```python
from build123d import *

# Parameters (mm, degrees)
SKETCH1_R           = 15
BOSS_EXTRUDE1_DEPTH = 850
SKETCH3_W           = 20
SKETCH3_H           = 50
BOSS_EXTRUDE2_DEPTH = 50


with BuildPart() as part:
    # Sketch1 → Boss-Extrude1 (new body)
    with BuildSketch(Plane.XY):
        Circle(SKETCH1_R)
    extrude(amount=BOSS_EXTRUDE1_DEPTH)

    # Sketch3 → Boss-Extrude2 (add)
    with BuildSketch(Plane.XY.offset(850)):
        Rectangle(SKETCH3_W, SKETCH3_H)
    boss_extrude2 = extrude(amount=BOSS_EXTRUDE2_DEPTH)

    # Mirror1: Boss-Extrude2 across plane
    add(boss_extrude2.mirror(Plane(origin=(0, 0, 425), x_dir=(1, 0, 0), z_dir=(0, 0, -1))))


solid = part.part
```
Input: part model. Units: mm. Frame: model coordinates. A direction names the side the tool comes from. Round coordinates to 2 decimals unless told otherwise and drop trailing zeros. Loops run counter-clockwise (first coordinate to the right, second up) from the corner with the lowest first, then second, coordinate; pieces in that order, holes last.
1) Pin query (flat end, axial travel): pin 1 (3 mm diameter, centred on x = 1, z = 82, fed in from -Y); pin 2 (1.5 mm diameter, centred on x = 13.5, y = 3.5, fed in from +Z); pin 3 (3 mm diameter, centred on y = -14.5, z = 597, fed in from +X). Return the tip coordinate at first contact, or that it passes through.
Ans:
pin 1: stops at y = -15
pin 2: stops at z = 850
pin 3: stops at x = 7.48
2) Section query C-C on z = 287. Return the cut outline in (x, y).
Ans:
outline: circle Ø30 at (0, 0)
3) Set-up query: faces 1 (the flat face through (-10, 0, 875)), 2 (the flat face through (10, 0, 875)), 3 (the flat face through (10, 0, -25)), 4 (the flat face through (0, 25, -25)). Return all of +Z, -Z, +X, -X, +Y, -Y with unobstructed straight access to the full face (end or side cutting, diameter ignored); none if empty.
Ans:
face 1: +Z, -X, +Y, -Y
face 2: +Z, +X, +Y, -Y
face 3: -Z, +X, +Y, -Y
face 4: +Z, -Z, +X, -X, +Y
4) Pull-direction query (Z, two-part tool) for faces 5 (the flat face through (0, 0, -50)), 6 (the flat face through (0, 0, 900)), 7 (the cylindrical face through (-14.985, 0.66, 419.05)), 8 (the flat face through (-10, 0, -25)); classes: released by +Z, released by -Z, zero draft, split by the parting line, or undercut.
Ans:
face 5: released by -Z
face 6: released by +Z
face 7: undercut
face 8: zero draft
5) Section query B-B on x = 0. Return the cut outline in (y, z), plus the area to 3 significant figures.
Ans:
outline: (-25, -50) - (25, -50) - (25, 0) - (15, 0) - (15, 850) - (25, 850) - (25, 900) - (-25, 900) - (-25, 850) - (-15, 850) - (-15, 0) - (-25, 0) - close
area: 30,500 mm2
6) Section query A-A on y = 0. Return the cut outline in (x, z), plus the area to 3 significant figures.
Ans:
outline: (-15, 0) - (-10, 0) - (-10, -50) - (10, -50) - (10, 0) - (15, 0) - (15, 850) - (10, 850) - (10, 900) - (-10, 900) - (-10, 850) - (-15, 850) - close
area: 27,500 mm2
7) Material intervals for line 1 (Z direction, x = -3, y = 15.5); line 2 (Y direction, x = 0.25, z = 693); line 3 (Z direction, x = -10.25, y = 9), sorted ascending.
Ans:
line 1: z = -50 to 0, 850 to 900
line 2: y = -15 to 15
line 3: z = 0 to 850
